Drawing for the job (mm, zero at the part's lowest x, y, z). A direction names the side the tool comes from. Round coordinates to 2 decimals unless told otherwise and drop trailing zeros. Order: outer loops, then holes, each group sorted by start corner. A loop starts at its lowest first (then second) coordinate and runs counter-clockwise, first axis right, second up. Notation, with made-up numbers: M 28.25,78.5 L 59.25,78.5 A22 cw 59.25,112.5 Z; hole C -36,-33 d2. An arc over 180 degrees is marked long. One line per item, written item: value. Start each with the question number.
Item 1: Probe L1, parallel to X at y = 3, z = 20; L2, parallel to Y at x = 26, z = 26. List the from-to ranges inside material, lowest first.
Item 2: Pin check, flat tips, straight feed: pin 1 (12 mm diameter, centred on x = 20.5, y = 55.5, fed in from +Z); pin 2 (2.5 mm diameter, centred on x = 35, z = 20, fed in from +Y); pin 3 (4.5 mm diameter, centred on x = 20, z = 35, fed in from +Y); pin 4 (8 mm diameter, centred on x = 16, y = 78.5, fed in from +Z). Stop position of each tip, or through.
Item 3: Tool access for the marked faces 1 and 2: list every direction of +Z, -Z, +X, -X, +Y, -Y with a clear straight run to the whole face (end or side of a thin tool).
Item 4: Band-saw the part on A-A, the plane x = 20. Write the cut outline in (y, z), then the cut area to 3 significant figures.
Item 5: Band-saw the part on D-D, the plane x = 35. Write the cut outline in (y, z).
Item 6: Band-saw the part on B-B, the plane z = 20. Write the cut outline in (x, y).
Item 7: Band-saw the part on C-C, the plane z = 35. Write the cut outline in (x, y).
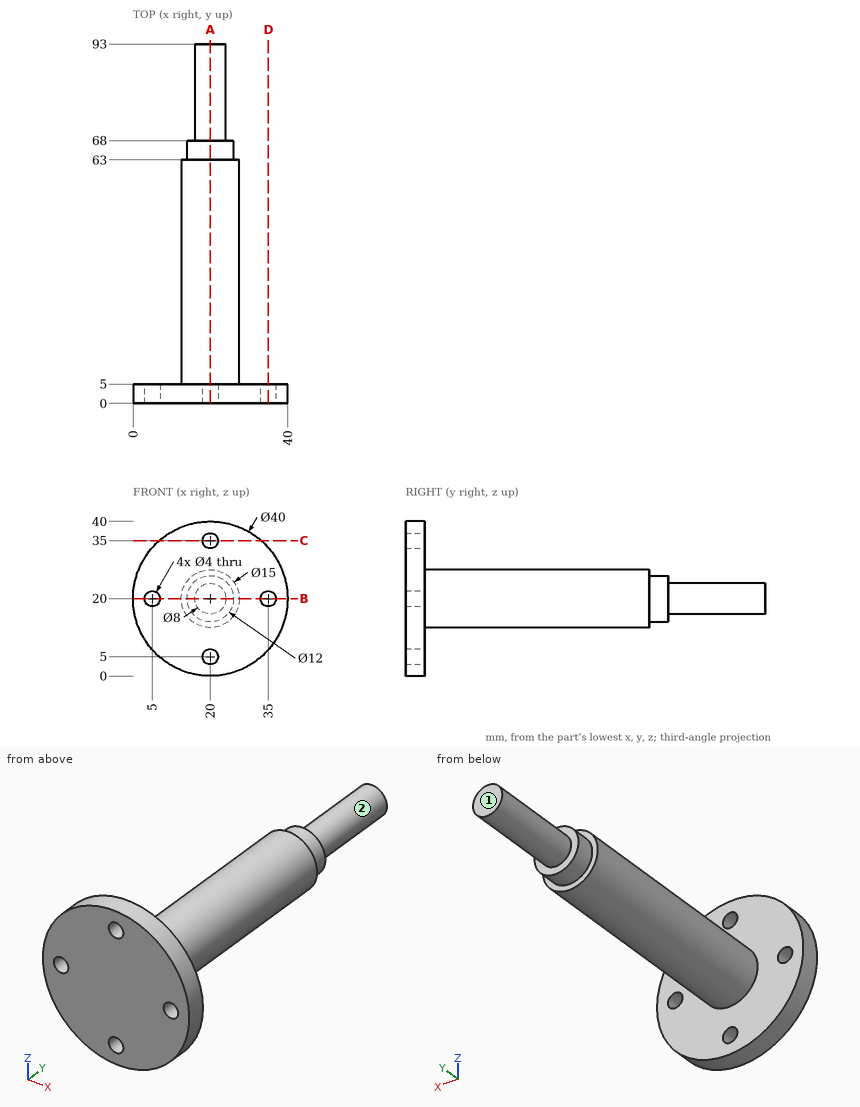
Output:
1. L1: x = 0 to 3, 7 to 33, 37 to 40
1. L2: y = 0 to 5
2. pin 1: stops at z = 27.5
2. pin 2: passes through
2. pin 3: stops at y = 5
2. pin 4: stops at z = 24
3. face 1: +Z, -Z, +X, -X, +Y
3. face 2: +Y
4. outline: M 0,0 L 5,0 L 5,3 L 0,3 Z; M 0,7 L 5,7 L 5,12.5 L 63,12.5 L 63,14 L 68,14 L 68,16 L 93,16 L 93,24 L 68,24 L 68,26 L 63,26 L 63,27.5 L 5,27.5 L 5,33 L 0,33 Z; M 0,37 L 5,37 L 5,40 L 0,40 Z
4. area: 1,290 mm²
5. outline: M 0,6.77 L 5,6.77 L 5,18 L 0,18 Z; M 0,22 L 5,22 L 5,33.23 L 0,33.23 Z
6. outline: M 0,0 L 3,0 L 3,5 L 0,5 Z; M 7,0 L 33,0 L 33,5 L 27.5,5 L 27.5,63 L 26,63 L 26,68 L 24,68 L 24,93 L 16,93 L 16,68 L 14,68 L 14,63 L 12.5,63 L 12.5,5 L 7,5 Z; M 37,0 L 40,0 L 40,5 L 37,5 Z
7. outline: M 6.77,0 L 18,0 L 18,5 L 6.77,5 Z; M 22,0 L 33.23,0 L 33.23,5 L 22,5 Z
